from build123d import *

# Parameters (mm, degrees)
F1_DEPTH = 57.15
F2_W     = 76.2
F2_H     = 50.960924
F3_DEPTH = 15.24


with BuildPart() as f1:
    # F0 (on Right) → F1 (new body, symmetric)
    with BuildSketch(Plane.YZ):
        Polygon((-76.2, 0), (0, 0), (0, 63.5), (-16.764, 63.5), (-31.75, 31.75), (-76.2, 31.75), align=None)
    extrude(amount=F1_DEPTH, both=True)

    # F2 (on face) → F3 (join)
    with BuildSketch(Plane.YZ.offset(57.15)):
        with Locations((-38.1, 25.480462)):
            Rectangle(F2_W, F2_H)
    extrude(amount=-F3_DEPTH)

    # F4: F1 across plane


with BuildPart() as f1_1:
    add(f1.part)
    add(f1.part.mirror(Plane.YZ))


solid = f1_1.part
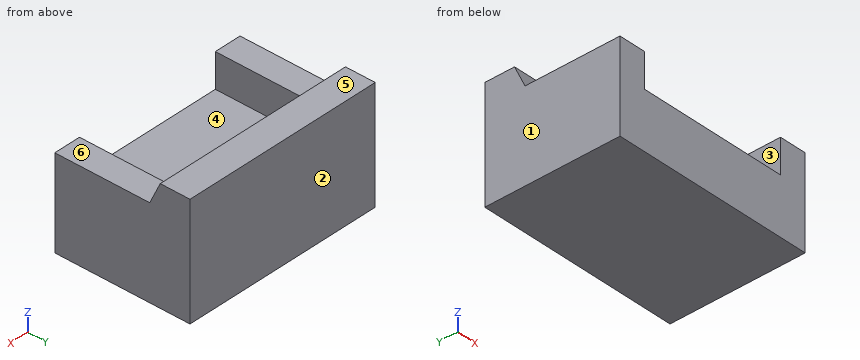
Build history of the part. All positions in model axes, mm. Face numbers are marked on the shaded views. A direction names the side the tool comes from. Round coordinates to 2 decimals unless told otherwise and drop trailing zeros. Write each loop counter-clockwise with the first axis right and the second up, starting at its lowest first coordinate (ties: lowest second). Pieces come first, ordered by that corner, then holes. Notation, with made-up numbers: (34, 34) -> (82, 34) arc R16 cw to (82, 39) -> close; hole circle Ø1 at (77, 64). An arc over 180 degrees is marked (long way). Write item = value, one per line.
(1) Band-saw the part on A-A (x = -23). Give the cut face in (y, z).
Answer:
outline = (-76.2, 0) -> (0, 0) -> (0, 63.5) -> (-16.76, 63.5) -> (-31.75, 31.75) -> (-76.2, 31.75) -> close
(2) Tool access for the marked faces 4, 5 and 6: list every direction of +Z, -Z, +X, -X, +Y, -Y with a clear straight run to the whole face (end or side of a thin tool).
Answer:
face_4 = +Z, -Y
face_5 = +Z, +X, -X, +Y, -Y
face_6 = +Z, +X, -X, -Y
(3) Flat gauge pins, fed straight in: pin 1 (2 mm diameter, centred on x = 20, y = -66.5, fed in from +Z); pin 2 (7.5 mm diameter, centred on x = 50, y = -51.5, fed in from +Z); pin 3 (1 mm diameter, centred on x = 33, z = 44.5, fed in from -Y). Where does each tip first touch, or does it go through?
Answer:
pin_1 = 31.75
pin_2 = 50.96
pin_3 = -25.97
(4) Band-saw the part on C-C (z = 35). Give the cut face in (x, y), then the cut area to 3 significant figures.
Answer:
outline = (-57.15, -76.2) -> (-41.91, -76.2) -> (-41.91, -30.22) -> (41.91, -30.22) -> (41.91, -76.2) -> (57.15, -76.2) -> (57.15, 0) -> (-57.15, 0) -> close
area = 4,860 mm2
(5) Probe L1, parallel to X at y = -43.5, z = 50.5; L2, parallel to Z at x = 43, y = -44; L3, parallel to Z at x = 35.5, y = -71.5. List the from-to ranges inside material, lowest first.
Answer:
L1 = -57.15 to -41.91, 41.91 to 57.15
L2 = 0 to 50.96
L3 = 0 to 31.75
(6) Band-saw the part on B-B (y = -63). Give the cut face in (x, z).
Answer:
outline = (-57.15, 0) -> (57.15, 0) -> (57.15, 50.96) -> (41.91, 50.96) -> (41.91, 31.75) -> (-41.91, 31.75) -> (-41.91, 50.96) -> (-57.15, 50.96) -> close
(7) Two-plate mould, pull along X, no slides. Class the marked faces 1, 2 and 3: pulls with the +X half, pulls with the -X half, needs draft (parallel to the pull), parting line crosses it, or undercut.
Answer:
face_1 = pulls with the -X half
face_2 = needs draft
face_3 = undercut
